from build123d import *

# Parameters (mm, degrees)
F0_W     = 46.0741333663
F0_H     = 38.6145105585
F1_DEPTH = 25
F2_DEPTH = 10
F3_R     = 10


with BuildPart() as f1:
    # F0 (on Top) → F1 (new body)
    with BuildSketch(Plane.XY):
        with Locations((-35.7623007149, 32.0324976929)):
            Rectangle(F0_W, F0_H)
    extrude(amount=F1_DEPTH)

    # F2 (add): a face of the model
    f2_faces = [f1.faces().sort_by_distance(p)[0] for p in [
        (-35.7623007149, 32.0324976929, 25),
    ]]
    extrude(f2_faces, amount=F2_DEPTH)

    # F3
    f3_edges = [f1.edges().sort_by_distance(p)[0] for p in [
        (-35.762301, 51.339753, 35),
        (-58.799367, 51.339753, 17.5),
        (-58.799367, 32.032498, 35),
        (-58.799367, 12.725242, 17.5),
        (-58.799367, 32.032498, 0),
        (-35.762301, 51.339753, 0),
        (-12.725234, 51.339753, 17.5),
        (-12.725234, 32.032498, 35),
        (-12.725234, 32.032498, 0),
        (-12.725234, 12.725242, 17.5),
        (-35.762301, 12.725242, 35),
        (-35.762301, 12.725242, 0),
    ]]
    fillet(f3_edges, radius=F3_R)


solid = f1.part
Work out the finished part from the listing and answer in its coordinate system (mm). Round coordinates to 2 decimals unless told otherwise and drop trailing zeros. Write each loop counter-clockwise with the first axis right and the second up, starting at its lowest first coordinate (ties: lowest second). Pieces come first, ordered by that corner, then holes.
1) A cutting plane is placed at A-A (z = 17). Give the vertices of the cut face in (x, y).
2) Straight lines are drawn through the part: line 1 (Z direction, x = -17, y = 16); line 2 (X direction, y = 42, z = 28); line 3 (Z direction, x = -26, y = 21.5). For each, find the intervals that lie inside material, in ascending order.
3) Given pin 1 Ø1.5 at (x, y) = (-52.5, 45.5) entering from +Z; pin 2 Ø5 at (x, z) = (-34, 6) entering from +Y; pin 3 Ø2 at (x, y) = (-53.5, 37.5) entering from -Z, each flat-ended and moving along its own axis, determine where each tip first touches the part or whether it passes through.
4) A cutting plane is placed at B-B (y = 26). Give the vertices of the cut face in (x, z), plus the area to 3 significant figures.
Completed:
1. outline: (-58.8, 22.73) arc R10 ccw to (-48.8, 12.73) - (-22.73, 12.73) arc R10 ccw to (-12.73, 22.73) - (-12.73, 41.34) arc R10 ccw to (-22.73, 51.34) - (-48.8, 51.34) arc R10 ccw to (-58.8, 41.34) - close
2. line 1: z = 5.31 to 29.69
2. line 2: x = -58.32 to -13.21
2. line 3: z = 0.08 to 34.92
3. pin 1: stops at z = 33.76
3. pin 2: stops at y = 51.23
3. pin 3: stops at z = 0.71
4. outline: (-58.8, 10) arc R10 ccw to (-48.8, 0) - (-22.73, 0) arc R10 ccw to (-12.73, 10) - (-12.73, 25) arc R10 ccw to (-22.73, 35) - (-48.8, 35) arc R10 ccw to (-58.8, 25) - close
4. area: 1,530 mm2
